```python
from build123d import *

# Parameters (mm, degrees)
F0_R     = 15
F1_DEPTH = 10
F2_R     = 20
F2_R_2   = 15
F3_DEPTH = 15
F4_R     = 2


with BuildPart() as f1:
    # F0 (on Top) → F1 (new body)
    with BuildSketch(Plane.XY):
        with BuildLine():
            Line((-25, -40), (25, -40))
            ThreePointArc((25, -40), (28.535534, -38.535534), (30, -35))
            Line((30, -35), (30, 35))
            ThreePointArc((30, 35), (28.535534, 38.535534), (25, 40))
            Line((25, 40), (-25, 40))
            ThreePointArc((-25, 40), (-28.535534, 38.535534), (-30, 35))
            Line((-30, 35), (-30, -35))
            ThreePointArc((-30, -35), (-28.535534, -38.535534), (-25, -40))
        make_face()
        Circle(F0_R, mode=Mode.SUBTRACT)
    extrude(amount=F1_DEPTH)

    # F2 (on face) → F3 (join)
    with BuildSketch(Plane.XY.offset(10)):
        Circle(F2_R)
        Circle(F2_R_2, mode=Mode.SUBTRACT)
    extrude(amount=F3_DEPTH)

    # F4
    f4_edges = [f1.edges().sort_by_distance(p)[0] for p in [
        (-20, 0, 25),
        (-15, 0, 25),
        (-28.535534, -38.535534, 10),
        (-30, 0, 10),
        (0, -40, 10),
        (-28.535534, 38.535534, 10),
        (28.535534, -38.535534, 10),
        (0, 40, 10),
        (30, 0, 10),
        (28.535534, 38.535534, 10),
        (-20, 0, 10),
    ]]
    fillet(f4_edges, radius=F4_R)


solid = f1.part
```
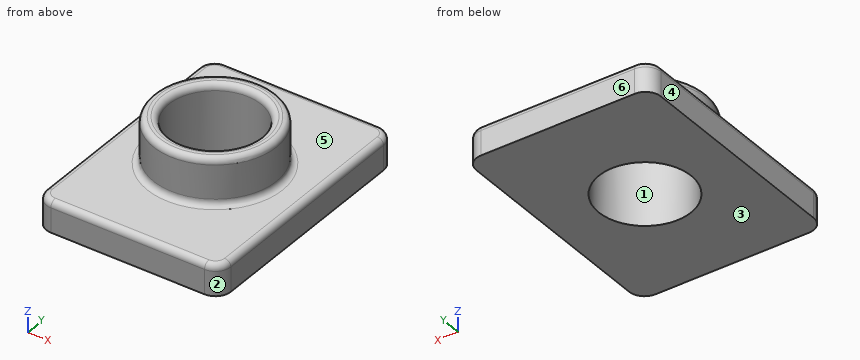
Verification items for the finished model (mm, model axes). Face numbers are marked on the shaded views. A direction names the side the tool comes from. Coordinates: 2 decimals unless noted, no trailing zeros. Loops run counter-clockwise (first coordinate to the right, second up) from the corner with the lowest first, then second, coordinate; pieces in that order, holes last. Notation, with made-up numbers: (29.5, 55.25) -> (33.5, 55.25) arc R16 ccw to (33.5, 59.25) -> close; hole circle Ø8 at (-25, 0.25). An arc over 180 degrees is marked (long way). Answer in a Markdown table with one row per item. Add a question column.
1. Material ranges on probe 1 along Y at (x, z) = (0, 6); probe 2 along Y at (x, z) = (0, 16.5); probe 3 along X at (y, z) = (-13, 9), recorded low to high. Write a range as [from, to].
2. Section check C-C, the plane z = 6.5. Enter the section's corners in (x, y).
3. Section check A-A, the plane y = 0. Enter the section's corners in (x, z), then the cut area to 3 significant figures.
4. Access from +Z, -Z, +X, -X, +Y, -Y to the whole of each face (thin tool, end or side, straight path). Record for the marked faces 5 and 6.
5. Section check B-B, the plane x = 0. Enter the section's corners in (y, z), then the cut area to 3 significant figures.
6. Section check D-D, the plane y = -30.5. Enter the section's corners in (x, z), then the cut area to 3 significant figures.
7. Draft check along X on the marked faces 1, 2, 3 and 4. Enter one of: +X half, -X half, draft (parallel to the pull), parting line (faces both ways), or undercut.
8. Depth check by flat-ended pin: P1, Ø8, axis at x = -20, y = 22, coming from the -Z side; P2, Ø8, axis at y = 32, z = 17.5, coming from the +X side; P3, Ø3, axis at x = 14, z = 11, coming from the +Y side; P4, Ø2, axis at x = -12.5, z = 15.5, coming from the -Y side. Enter the tip coordinate at first touch or a pass-through.
Derived:
| question | item | result |
|---|---|---|
| 1 | probe 1 | y = [-40, -15], [15, 40] |
| 1 | probe 2 | y = [-20, -15], [15, 20] |
| 1 | probe 3 | x = [-29.73, -7.48], [7.48, 29.73] |
| 2 | outline | (-30, -35) arc R5 ccw to (-25, -40) -> (25, -40) arc R5 ccw to (30, -35) -> (30, 35) arc R5 ccw to (25, 40) -> (-25, 40) arc R5 ccw to (-30, 35) -> close; hole circle Ø30 at (0, 0) |
| 3 | outline | (-30, 0) -> (-15, 0) -> (-15, 23) arc R2 ccw to (-17, 25) -> (-18, 25) arc R2 ccw to (-20, 23) -> (-20, 12) arc R2 cw to (-22, 10) -> (-28, 10) arc R2 ccw to (-30, 8) -> close; (15, 0) -> (30, 0) -> (30, 8) arc R2 ccw to (28, 10) -> (22, 10) arc R2 cw to (20, 12) -> (20, 23) arc R2 ccw to (18, 25) -> (17, 25) arc R2 ccw to (15, 23) -> close |
| 3 | area | 447 mm² |
| 4 | face 5 | +Z |
| 4 | face 6 | +Z, -Z, +X, -X, +Y |
| 5 | outline | (-40, 0) -> (-15, 0) -> (-15, 23) arc R2 ccw to (-17, 25) -> (-18, 25) arc R2 ccw to (-20, 23) -> (-20, 12) arc R2 cw to (-22, 10) -> (-38, 10) arc R2 ccw to (-40, 8) -> close; (15, 0) -> (40, 0) -> (40, 8) arc R2 ccw to (38, 10) -> (22, 10) arc R2 cw to (20, 12) -> (20, 23) arc R2 ccw to (18, 25) -> (17, 25) arc R2 ccw to (15, 23) -> close |
| 5 | area | 647 mm² |
| 6 | outline | (-30, 0) -> (30, 0) -> (30, 8) arc R2 ccw to (28, 10) -> (-28, 10) arc R2 ccw to (-30, 8) -> close |
| 6 | area | 598 mm² |
| 7 | face 1 | undercut |
| 7 | face 2 | +X half |
| 7 | face 3 | draft |
| 7 | face 4 | -X half |
| 8 | P1 | stops at z = 0 |
| 8 | P2 | passes through |
| 8 | P3 | stops at y = 39.32 |
| 8 | P4 | stops at y = -16.36 |
